Here's how the part is built. I have some questions about the finished solid (model axes, mm). Face numbers are marked on the shaded views. A direction names the side the tool comes from. Give positions to 0.01 mm unless a question says otherwise; leave off trailing zeros. Loops run counter-clockwise (first coordinate to the right, second up) from the corner with the lowest first, then second, coordinate; pieces in that order, holes last. Notation, with made-up numbers: M 20,4 L 24,4 A24 cw 24,34 Z; hole C 52.25,-23.5 d9. An arc over 180 degrees is marked long. Answer as CSV lines item,"result". Start each with the question number.
Item 1: If I drill on line 1 along Z through (x, y) = (25, -3.5); line 2 along X through (y, z) = (-18.25, 32.5); line 3 along X through (y, z) = (-14, 22.5), over which ranges is the centre line in solid material (lowest first)? Write a range as from..to.
Item 2: I want a section at A-A on y = -3.5. List the corners of the cut face in (x, z) for me, plus the area to 3 significant figures.
Item 3: For the marked faces 1 and 2, which set-ups out of +Z, -Z, +X, -X, +Y, -Y let a thin tool reach every point of the face, with its end or its side?
Item 4: I want a section at B-B on x = 23. List the corners of the cut face in (y, z) for me.
Item 5: I want a section at C-C on z = 23. List the corners of the cut face in (x, y) for me.
Item 6: Will these pins go through, and if not, where does the flat tip stop? P1, Ø3, axis at x = 22, y = -8.5, coming from the +Z side; P2, Ø2, axis at y = -6, z = 15.5, coming from the +X side.
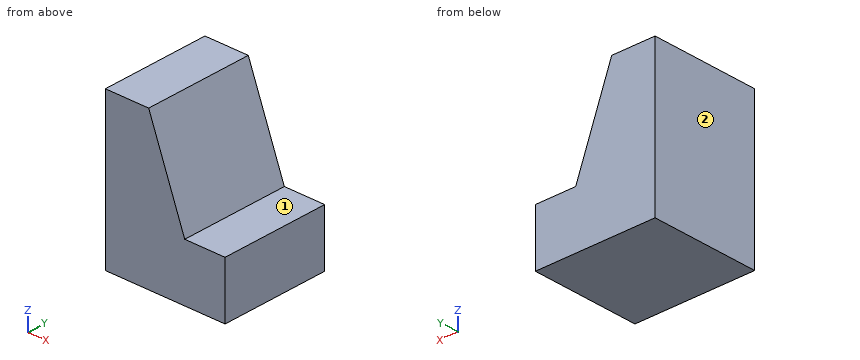
from build123d import *

# Parameters (mm, degrees)
F0_W     = 37.4921225011
F0_H     = 35.8838811517
F1_DEPTH = 25.4
F3_DEPTH = 25.4
F4_W     = 9.4484174624
F4_H     = 13.1674753502
F5_DEPTH = 25.4


with BuildPart() as f1:
    # F0 (on Front) → F1 (new body)
    with BuildSketch(Plane.XZ):
        with Locations((18.7460612506, 17.9419405758)):
            Rectangle(F0_W, F0_H)
    extrude(amount=F1_DEPTH)

    # F2 (on face) → F3 (cut)
    with BuildSketch(Plane.XZ.offset(25.4)):
        Polygon((37.4921225011, 35.8838811517), (10.1520223543, 35.8838811517), (18.5952875763, 13.1674753502), (37.4921225011, 13.1674753502), align=None)
    extrude(amount=-F3_DEPTH, mode=Mode.SUBTRACT)

    # F4 (on face) → F5 (cut)
    with BuildSketch(Plane.XZ.offset(25.4)):
        with Locations((32.7679137699, 6.5837376751)):
            Rectangle(F4_W, F4_H)
    extrude(amount=-F5_DEPTH, mode=Mode.SUBTRACT)


solid = f1.part
Result:
1,line 1,"0..13.17"
1,line 2,"0..11.41"
1,line 3,"0..15.13"
2,outline,"M 0,0 L 28.04,0 L 28.04,13.17 L 18.6,13.17 L 10.15,35.88 L 0,35.88 Z"
2,area,"696 mm^2"
3,face 1,"+Z, +X, +Y, -Y"
3,face 2,"+Z, -Z, -X, +Y, -Y"
4,outline,"M -25.4,0 L 0,0 L 0,13.17 L -25.4,13.17 Z"
5,outline,"M 0,-25.4 L 14.94,-25.4 L 14.94,0 L 0,0 Z"
6,P1,"z = 13.17"
6,P2,"x = 18.1"
